Autodesk Inventor part; units mm, degrees
ref_plane "YZ Plane" through (0, 0, 0) normal (1, 0, 0) x (0, 1, 0)
ref_plane "XZ Plane" through (0, 0, 0) normal (0, 1, 0) x (-1, 0, 0)
ref_plane "XY Plane" through (0, 0, 0) normal (0, 0, 1) x (1, 0, 0)
sketch "Sketch1" plane through (0, 0, 0) normal (0, 1, 0) x (-1, 0, 0)
  circle A0 centre (0, 0) radius 17
  circle A1 centre (0, 0) radius 13.845
  circle A2 centre (17, 0) radius 1.075
  line L0 (19.2, 2.875) -> (14.8, 2.875)
  line L1 (14.8, 2.875) -> (14.8, -2.875)
  line L2 (14.8, -2.875) -> (19.2, -2.875)
  line L3 (19.2, -2.875) -> (19.2, 2.875)
  line L4 (19.2, 2.875) -> (14.8, -2.875) construction
  line L5 (14.8, 2.875) -> (19.2, -2.875) construction
  circle A3 centre (12.0208, 12.0208) radius 1.075
  line L6 (11.5435, 15.6094) -> (8.4322, 12.4981)
  line L7 (8.4322, 12.4981) -> (12.4981, 8.4322)
  line L8 (12.4981, 8.4322) -> (15.6094, 11.5435)
  line L9 (15.6094, 11.5435) -> (11.5435, 15.6094)
  line L10 (11.5435, 15.6094) -> (12.4981, 8.4322) construction
  line L11 (8.4322, 12.4981) -> (15.6094, 11.5435) construction
  circle A4 centre (0, 17) radius 1.075
  line L12 (-2.875, 19.2) -> (-2.875, 14.8)
  line L13 (-2.875, 14.8) -> (2.875, 14.8)
  line L14 (2.875, 14.8) -> (2.875, 19.2)
  line L15 (2.875, 19.2) -> (-2.875, 19.2)
  line L16 (-2.875, 19.2) -> (2.875, 14.8) construction
  line L17 (-2.875, 14.8) -> (2.875, 19.2) construction
  circle A5 centre (-12.0208, 12.0208) radius 1.075
  line L18 (-15.6094, 11.5435) -> (-12.4981, 8.4322)
  line L19 (-12.4981, 8.4322) -> (-8.4322, 12.4981)
  line L20 (-8.4322, 12.4981) -> (-11.5435, 15.6094)
  line L21 (-11.5435, 15.6094) -> (-15.6094, 11.5435)
  line L22 (-15.6094, 11.5435) -> (-8.4322, 12.4981) construction
  line L23 (-12.4981, 8.4322) -> (-11.5435, 15.6094) construction
  circle A6 centre (-17, 0) radius 1.075
  line L24 (-19.2, -2.875) -> (-14.8, -2.875)
  line L25 (-14.8, -2.875) -> (-14.8, 2.875)
  line L26 (-14.8, 2.875) -> (-19.2, 2.875)
  line L27 (-19.2, 2.875) -> (-19.2, -2.875)
  line L28 (-19.2, -2.875) -> (-14.8, 2.875) construction
  line L29 (-14.8, -2.875) -> (-19.2, 2.875) construction
  circle A7 centre (-12.0208, -12.0208) radius 1.075
  line L30 (-11.5435, -15.6094) -> (-8.4322, -12.4981)
  line L31 (-8.4322, -12.4981) -> (-12.4981, -8.4322)
  line L32 (-12.4981, -8.4322) -> (-15.6094, -11.5435)
  line L33 (-15.6094, -11.5435) -> (-11.5435, -15.6094)
  line L34 (-11.5435, -15.6094) -> (-12.4981, -8.4322) construction
  line L35 (-8.4322, -12.4981) -> (-15.6094, -11.5435) construction
  circle A8 centre (0, -17) radius 1.075
  line L36 (2.875, -19.2) -> (2.875, -14.8)
  line L37 (2.875, -14.8) -> (-2.875, -14.8)
  line L38 (-2.875, -14.8) -> (-2.875, -19.2)
  line L39 (-2.875, -19.2) -> (2.875, -19.2)
  line L40 (2.875, -19.2) -> (-2.875, -14.8) construction
  line L41 (2.875, -14.8) -> (-2.875, -19.2) construction
  circle A9 centre (12.0208, -12.0208) radius 1.075
  line L42 (15.6094, -11.5435) -> (12.4981, -8.4322)
  line L43 (12.4981, -8.4322) -> (8.4322, -12.4981)
  line L44 (8.4322, -12.4981) -> (11.5435, -15.6094)
  line L45 (11.5435, -15.6094) -> (15.6094, -11.5435)
  line L46 (15.6094, -11.5435) -> (8.4322, -12.4981) construction
  line L47 (12.4981, -8.4322) -> (11.5435, -15.6094) construction
  point P0 (16.7551, 2.875)
  point P1 (13.8806, 9.8147)
  point P2 (9.8147, 13.8806)
  point P3 (2.875, 16.7551)
  point P4 (-2.875, 16.7551)
  point P5 (-9.8147, 13.8806)
  point P6 (-13.8806, 9.8147)
  point P7 (-16.7551, 2.875)
  point P8 (-16.7551, -2.875)
  point P9 (-13.8806, -9.8147)
  point P10 (-9.8147, -13.8806)
  point P11 (-2.875, -16.7551)
  point P12 (2.875, -16.7551)
  point P13 (9.8147, -13.8806)
  point P14 (13.8806, -9.8147)
  point P15 (16.7551, -2.875)
  dimension "d0" = 34
  dimension "d1" = 27.69
  dimension "d2" = 5.75
  dimension "d3" = 2.15
  dimension "d4" = 4.4
  dimension "d7" = 360
extrude "Extrusion1" add sketch "Sketch1" along normal blind 5.5 contours A2 A0 L2 L1 L0 | A0 L0 L3 L2 A2 | L0 L1 L2 A0 L42 L43 L44 L36 L37 L38 L30 L31 L32 L24 L25 L26 L18 L19 L20 L12 L13 L14 L6 L7 L8 | L8 L7 L6 A0 A3 | A0 A3 L6 L9 L8 | L42 L45 L44 A0 A9 | A0 A9 L44 L43 L42 | L14 L13 L12 A0 A4 | A0 A4 L12 L15 L14 | L36 L39 L38 A0 A8 | A0 A8 L38 L37 L36 | L20 L19 L18 A0 A5 | A0 A5 L18 L21 L20 | L30 L33 L32 A0 A7 | A0 A7 L32 L31 L30 | L26 L25 L24 A0 A6 | A0 A6 L24 L27 L26
properties part number "24vFastener"
Could you check a few things on this model? Use its own coordinates, in mm. A direction names the side the tool comes from. Give positions to 0.01 mm unless a question says otherwise; leave off trailing zeros. Order: outer loops, then holes, each group sorted by start corner. A loop starts at its lowest first (then second) coordinate and runs counter-clockwise, first axis right, second up. Notation, with made-up numbers: (-14, -20) -> (9, -20) arc R32 cw to (9, 14) -> close; hole circle Ø8 at (78.25, 62.5). An arc over 180 degrees is marked (long way). Answer in a Markdown table with one row per item. Add a question column.
Item 1: Imagine slicing it at B-B (z = 10.5). List the corners of the cut face in (x, y) for me, and give its area (3 significant figures).
Item 2: Imagine slicing it at D-D (x = 15). List the corners of the cut face in (y, z) for me.
Item 3: We'd pull the mould along X, two halves only. Please class faces 5 (the flat face through (18, 3, 2.875)), 6 (the cylindrical face through (0.14, 2.712, 15.934)), 7 (the flat face through (-13.605, 2.712, 13.548)), 8 (the flat face through (2.875, 3, -18)): pulls with the +X half, pulls with the -X half, needs draft (parallel to the pull), parting line crosses it, or undercut.
Item 4: For faces 1 (the flat face through (-2.875, 3, 18)), 2 (the flat face through (2.875, 3, 18)), 3 (the flat face through (18, 3, -2.875)), 4 (the cylindrical face through (-15.726, 2.712, -6.457)), which set-ups out of +Z, -Z, +X, -X, +Y, -Y let a thin tool reach every point of the face, with its end or its side?
Item 5: I'm going to push flat-ended pins straight in: P1, Ø10, axis at x = 8.5, z = 0, coming from the -Y side; P2, Ø1.2, axis at x = -18, y = 1.5, coming from the +Z side (3 decimals); P3, Ø3, axis at y = 4.5, z = -13.5, coming from the +X side; P4, Ø1.2, axis at y = 1.5, z = -17.5, coming from the -X side (3 decimals). Where does each tip first touch, or does it pass through?
Item 6: Please list where these lines run through material, in increasing order: probe 1 along Z at (x, y) = (-17, 1.95) (3 decimals); probe 2 along Z at (x, y) = (15, 1.3); probe 3 along Z at (x, y) = (-5, 4.45).
Item 7: Imagine slicing it at C-C (z = -0.5). List the corners of the cut face in (x, y) for me, and give its area (3 significant figures).
Item 8: Imagine slicing it at A-A (x = 0). List the corners of the cut face in (y, z) for me (3 decimals).
Result:
| question | item | result |
|---|---|---|
| 1 | outline | (-14.57, 0) -> (-9.02, 0) -> (-9.02, 5.5) -> (-14.57, 5.5) -> close; (9.02, 0) -> (14.57, 0) -> (14.57, 5.5) -> (9.02, 5.5) -> close |
| 1 | area | 61.0 mm2 |
| 2 | outline | (0, -12.15) -> (5.5, -12.15) -> (5.5, -10.93) -> (0, -10.93) -> close; (0, -8) -> (5.5, -8) -> (5.5, 8) -> (0, 8) -> close; (0, 10.93) -> (5.5, 10.93) -> (5.5, 12.15) -> (0, 12.15) -> close |
| 3 | face 5 | needs draft |
| 3 | face 6 | undercut |
| 3 | face 7 | pulls with the -X half |
| 3 | face 8 | pulls with the +X half |
| 4 | face 1 | +Z, -X, +Y, -Y |
| 4 | face 2 | +Z, +X, +Y, -Y |
| 4 | face 3 | -Z, +X, +Y, -Y |
| 4 | face 4 | -X, +Y, -Y |
| 5 | P1 | through |
| 5 | P2 | z = 2.875 |
| 5 | P3 | x = 15.15 |
| 5 | P4 | x = -2.875 |
| 6 | probe 1 | -2.875 to -1.075, 1.075 to 2.875 |
| 6 | probe 2 | -12.15 to -10.93, -8 to 8, 10.93 to 12.15 |
| 6 | probe 3 | -16.25 to -12.91, 12.91 to 16.25 |
| 7 | outline | (-19.2, 0) -> (-17.95, 0) -> (-17.95, 5.5) -> (-19.2, 5.5) -> close; (-16.05, 0) -> (-13.84, 0) -> (-13.84, 5.5) -> (-16.05, 5.5) -> close; (13.84, 0) -> (16.05, 0) -> (16.05, 5.5) -> (13.84, 5.5) -> close; (17.95, 0) -> (19.2, 0) -> (19.2, 5.5) -> (17.95, 5.5) -> close |
| 7 | area | 38.1 mm2 |
| 8 | outline | (0, -19.2) -> (5.5, -19.2) -> (5.5, -18.075) -> (0, -18.075) -> close; (0, -15.925) -> (5.5, -15.925) -> (5.5, -13.845) -> (0, -13.845) -> close; (0, 13.845) -> (5.5, 13.845) -> (5.5, 15.925) -> (0, 15.925) -> close; (0, 18.075) -> (5.5, 18.075) -> (5.5, 19.2) -> (0, 19.2) -> close |
